Design review of the part shown in the three views and the two pictorial views. Dimensions are in mm from the part's minimum x, y and z. Coordinates: 2 decimals unless noted, no trailing zeros. Loops run counter-clockwise (first coordinate to the right, second up) from the corner with the lowest first, then second, coordinate; pieces in that order, holes last. Notation, with made-up numbers: (6.5, 25.25) -> (50.5, 25.25) arc R24 cw to (50.5, 62.25) -> close; hole circle Ø4 at (14.25, -16). An arc over 180 degrees is marked (long way). Answer in a Markdown table with one row per item.
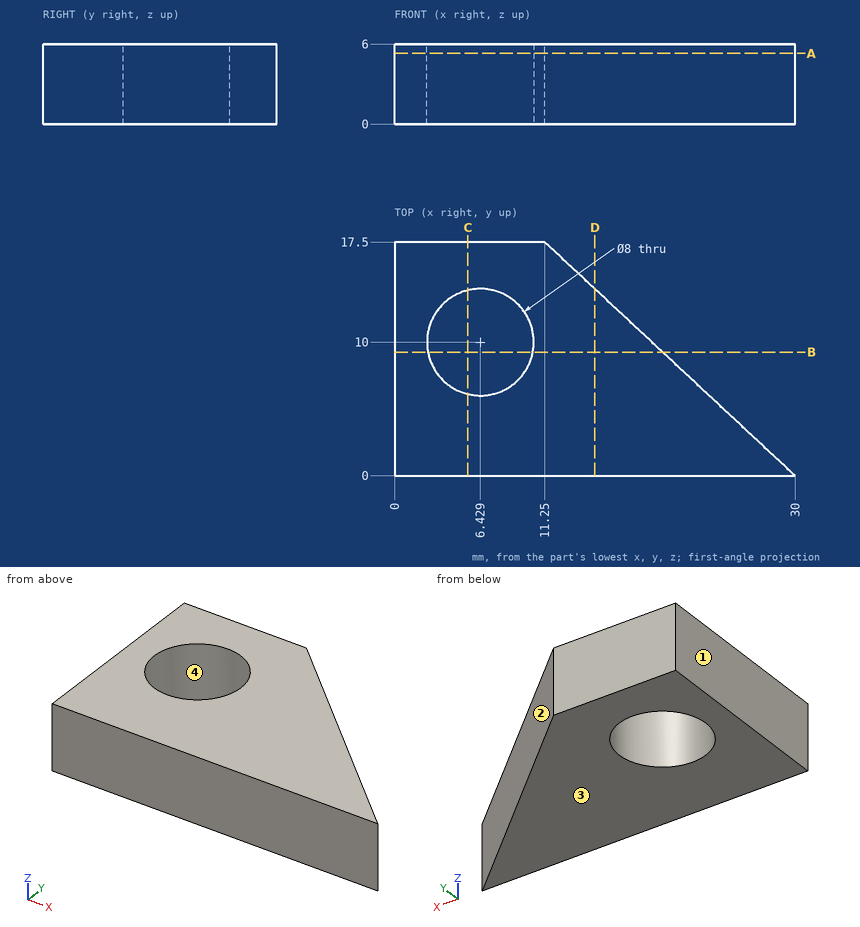
Item 1: Take a section at A-A, the plane z = 5.3. State the section outline as (x, y) points, and give its area (3 significant figures).
Worked answers:
| item | result |
|---|---|
| outline | (0, 0) -> (30, 0) -> (11.25, 17.5) -> (0, 17.5) -> close; hole circle Ø8 at (6.43, 10) |
| area | 311 mm² |
Item 2: Take a section at C-C, the plane x = 5.5. State the section outline as (y, z) points, and give its area (3 significant figures).
Worked answers:
| item | result |
|---|---|
| outline | (0, 0) -> (6.11, 0) -> (6.11, 6) -> (0, 6) -> close; (13.89, 0) -> (17.5, 0) -> (17.5, 6) -> (13.89, 6) -> close |
| area | 58.3 mm² |
Item 3: For L1, parallel to Y at x = 6.5, z = 4.9; L2, parallel to X at y = 8.5, z = 2.35 (1 decimal); L3, parallel to Y at x = 4.5, z = 1.2 (1 decimal), list the stretches that pass through material, from the lowest coordinate up.
Worked answers:
| item | result |
|---|---|
| L1 | 0 to 6, 14 to 17.5 |
| L2 | 0 to 2.7, 10.1 to 20.9 |
| L3 | 0 to 6.5, 13.5 to 17.5 |
Item 4: The part is to be moulded in two halves that separate along X. For the marked faces 1, 2, 3 and 4, say which applies: +X half, -X half, draft (parallel to the pull), parting line (faces both ways), or undercut.
Worked answers:
| item | result |
|---|---|
| face 1 | -X half |
| face 2 | +X half |
| face 3 | draft |
| face 4 | undercut |
Item 5: Take a section at D-D, the plane x = 15. State the section outline as (y, z) points.
Worked answers:
| item | result |
|---|---|
| outline | (0, 0) -> (14, 0) -> (14, 6) -> (0, 6) -> close |
Item 6: Insertion check: pin 1 (3 mm diameter, centred on x = 23, y = 10, fed in from -Z); pin 2 (1.5 mm diameter, centred on y = 10.5, z = 2.5, fed in from +X) (1 decimal). Each pin has a flat end and moves straight along its axis. Give the tip position at first contact, or say it passes through.
Worked answers:
| item | result |
|---|---|
| pin 1 | through |
| pin 2 | x = 19.6 |
Item 7: Take a section at B-B, the plane y = 9.25. State the section outline as (x, z) points.
Worked answers:
| item | result |
|---|---|
| outline | (0, 0) -> (2.5, 0) -> (2.5, 6) -> (0, 6) -> close; (10.36, 0) -> (20.09, 0) -> (20.09, 6) -> (10.36, 6) -> close |
